Work out the finished part from the listing and answer in its coordinate system (mm). Coordinates: 2 decimals unless noted, no trailing zeros. Order: outer loops, then holes, each group sorted by start corner. A loop starts at its lowest first (then second) coordinate and runs counter-clockwise, first axis right, second up.
```python
from build123d import *

# Parameters (mm, degrees)
F1_DEPTH = 12.7


with BuildPart() as f1:
    # F0 (on Right) → F1 (new body)
    with BuildSketch(Plane.YZ):
        Polygon((50.8, 292.1), (50.8, 304.8), (25.4, 304.8), (25.4, 292.1), (0, 292.1), (0, 304.8), (-25.4, 304.8), (-25.4, 292.1), (-50.8, 292.1), (-50.8, 304.8), (-76.2, 304.8), (-76.2, -304.8), (-50.8, -304.8), (-50.8, -292.1), (-25.4, -292.1), (-25.4, -304.8), (0, -304.8), (0, -292.1), (25.4, -292.1), (25.4, -304.8), (50.8, -304.8), (50.8, -292.1), (76.2, -292.1), (76.2, 292.1), align=None)
    extrude(amount=F1_DEPTH)


solid = f1.part
```
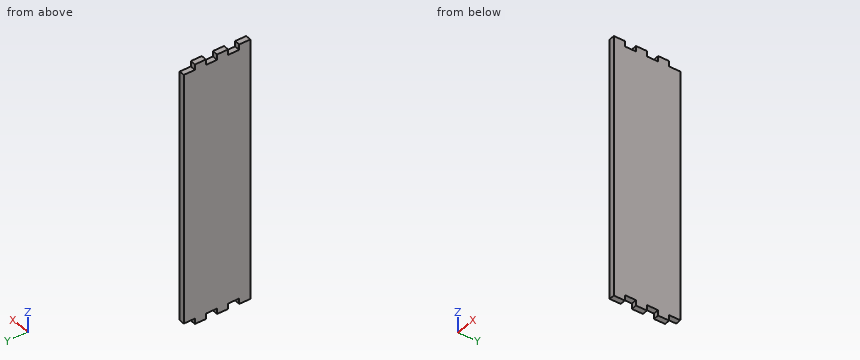
1. The part is cut by section B-B (y = -33.5). Determine the outline of the cut face in (x, z).
2. Consider probe 1 along Z at (x, y) = (6.5, 14.5). Determine where the line is inside the solid, lowest interval first.
3. Flat-ended cylindrical pins translate along their axes: pin 1 (4 mm diameter, centred on x = 6, z = 300.5, fed in from +Y); pin 2 (4 mm diameter, centred on x = 4, y = -43, fed in from -Z); pin 3 (1.5 mm diameter, centred on x = 1.5, y = 12, fed in from +Z). Find the tip coordinate at first contact, or state that the pin passes through.
4. The part is cut by section A-A (x = 7). Determine the outline of the cut face in (y, z), plus the area to 3 significant figures.
Worked out:
1. outline: (0, -292.1) - (12.7, -292.1) - (12.7, 292.1) - (0, 292.1) - close
2. probe 1: z = -292.1 to 292.1
3. pin 1: stops at y = 50.8
3. pin 2: stops at z = -292.1
3. pin 3: stops at z = 292.1
4. outline: (-76.2, -304.8) - (-50.8, -304.8) - (-50.8, -292.1) - (-25.4, -292.1) - (-25.4, -304.8) - (0, -304.8) - (0, -292.1) - (25.4, -292.1) - (25.4, -304.8) - (50.8, -304.8) - (50.8, -292.1) - (76.2, -292.1) - (76.2, 292.1) - (50.8, 292.1) - (50.8, 304.8) - (25.4, 304.8) - (25.4, 292.1) - (0, 292.1) - (0, 304.8) - (-25.4, 304.8) - (-25.4, 292.1) - (-50.8, 292.1) - (-50.8, 304.8) - (-76.2, 304.8) - close
4. area: 91,000 mm2
